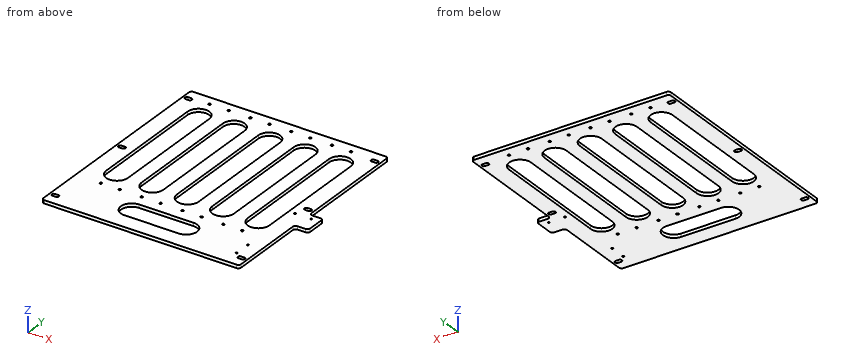
from build123d import *

# Parameters (mm, degrees)
SKETCH_1_W             = 363
SKETCH_1_H             = 403
EXTRUDE_1_DEPTH        = 6
FILLET_1_R             = 5
SKETCH_3_R             = 3.5
CUT_EXTRUDE_2_DEPTH    = 10
HOLE_WIZARD_M5_1_D     = 4.2
HOLE_WIZARD_M5_1_DEPTH = 12.4
HOLE_WIZARD_M5_1_TIP   = 1.2618073
CUT_EXTRUDE_3_DEPTH    = 10
CUT_EXTRUDE_4_DEPTH    = 10
CUT_EXTRUDE_5_DEPTH    = 10
HOLE_WIZARD_M4_1_D     = 3.3
HOLE_WIZARD_M4_1_DEPTH = 10.1
HOLE_WIZARD_M4_1_TIP   = 0.991420021
SKETCH_11_W            = 25
SKETCH_11_H            = 40
EXTRUDE_2_DEPTH        = 6
HOLE_WIZARD_M4_2_D     = 3.3
HOLE_WIZARD_M4_2_DEPTH = 10.1
HOLE_WIZARD_M4_2_TIP   = 0.991420021
FILLET_2_R             = 5


with BuildPart() as part:
    # Sketch 1 → 凸台-拉伸1 (new body)
    with BuildSketch(Plane.XY):
        Rectangle(SKETCH_1_W, SKETCH_1_H)
    extrude(amount=EXTRUDE_1_DEPTH)

    # 圆角1
    fillet_1_edges = [part.edges().sort_by_distance(p)[0] for p in [
        (181.5, -201.5, 3),
        (-181.5, -201.5, 3),
        (-181.5, 201.5, 3),
        (181.5, 201.5, 3),
    ]]
    fillet(fillet_1_edges, radius=FILLET_1_R)

    # 草图3 → 切除-拉伸2 (cut)
    with BuildSketch(Plane.XY.offset(6)):
        with Locations((-171, -180)):
            Circle(SKETCH_3_R)
        with Locations((-171, 180)):
            Circle(SKETCH_3_R)
        with Locations((-171, 0)):
            Circle(SKETCH_3_R)
        with Locations((171, 0)):
            Circle(SKETCH_3_R)
        with Locations((171, 180)):
            Circle(SKETCH_3_R)
        with Locations((171, -180)):
            Circle(SKETCH_3_R)
    extrude(amount=-CUT_EXTRUDE_2_DEPTH, mode=Mode.SUBTRACT)

    # M5 螺纹孔1
    with Locations(Plane.XY.offset(6)):
        with Locations((-135, -110), (-100, -110), (-135, 184), (-100, 184), (-60, -110), (-25, -110), (-60, 184), (-25, 184), (15, -110), (50, -110), (15, 184), (50, 184), (90, -110), (125, -110), (90, 184), (125, 184)):
            Hole(HOLE_WIZARD_M5_1_D / 2, depth=HOLE_WIZARD_M5_1_DEPTH)
            with Locations((0, 0, -(HOLE_WIZARD_M5_1_DEPTH + HOLE_WIZARD_M5_1_TIP / 2))):  # 118° drill point
                Cone(0, HOLE_WIZARD_M5_1_D / 2, HOLE_WIZARD_M5_1_TIP, mode=Mode.SUBTRACT)

    # 草图6 → 切除-拉伸3 (cut)
    with BuildSketch(Plane.XY.offset(6)):
        with BuildLine():
            Line((-174, 183.5), (-168, 183.5))
            ThreePointArc((-168, 183.5), (-164.5, 180), (-168, 176.5))
            Line((-168, 176.5), (-174, 176.5))
            ThreePointArc((-174, 176.5), (-177.5, 180), (-174, 183.5))
        make_face()
        with BuildLine():
            Line((168, 183.5), (174, 183.5))
            ThreePointArc((174, 183.5), (177.5, 180), (174, 176.5))
            Line((174, 176.5), (168, 176.5))
            ThreePointArc((168, 176.5), (164.5, 180), (168, 183.5))
        make_face()
        with BuildLine():
            Line((168, 3.5), (174, 3.5))
            ThreePointArc((174, 3.5), (177.5, 0), (174, -3.5))
            Line((174, -3.5), (168, -3.5))
            ThreePointArc((168, -3.5), (164.5, 0), (168, 3.5))
        make_face()
        with BuildLine():
            Line((168, -176.5), (174, -176.5))
            ThreePointArc((174, -176.5), (177.5, -180), (174, -183.5))
            Line((174, -183.5), (168, -183.5))
            ThreePointArc((168, -183.5), (164.5, -180), (168, -176.5))
        make_face()
        with BuildLine():
            Line((-174, 3.5), (-168, 3.5))
            ThreePointArc((-168, 3.5), (-164.5, 0), (-168, -3.5))
            Line((-168, -3.5), (-174, -3.5))
            ThreePointArc((-174, -3.5), (-177.5, 0), (-174, 3.5))
        make_face()
        with BuildLine():
            Line((-174, -176.5), (-168, -176.5))
            ThreePointArc((-168, -176.5), (-164.5, -180), (-168, -183.5))
            Line((-168, -183.5), (-174, -183.5))
            ThreePointArc((-174, -183.5), (-177.5, -180), (-174, -176.5))
        make_face()
    extrude(amount=-CUT_EXTRUDE_3_DEPTH, mode=Mode.SUBTRACT)

    # 草图7 → 切除-拉伸4 (cut)
    with BuildSketch(Plane.XY.offset(6)):
        with BuildLine():
            Line((-50, -131.5), (50, -131.5))
            ThreePointArc((50, -131.5), (70, -151.5), (50, -171.5))
            Line((50, -171.5), (-50, -171.5))
            ThreePointArc((-50, -171.5), (-70, -151.5), (-50, -131.5))
        make_face()
    extrude(amount=-CUT_EXTRUDE_4_DEPTH, mode=Mode.SUBTRACT)

    # 草图8 → 切除-拉伸5 (cut)
    with BuildSketch(Plane.XY.offset(6)):
        with BuildLine():
            Line((20, 146.5), (20, -73.5))
            ThreePointArc((20, -73.5), (0, -93.5), (-20, -73.5))
            Line((-20, -73.5), (-20, 146.5))
            ThreePointArc((-20, 146.5), (0, 166.5), (20, 146.5))
        make_face()
        with BuildLine():
            Line((85, 146.5), (85, -73.5))
            ThreePointArc((85, -73.5), (65, -93.5), (45, -73.5))
            Line((45, -73.5), (45, 146.5))
            ThreePointArc((45, 146.5), (65, 166.5), (85, 146.5))
        make_face()
        with BuildLine():
            Line((150, 146.5), (150, -73.5))
            ThreePointArc((150, -73.5), (130, -93.5), (110, -73.5))
            Line((110, -73.5), (110, 146.5))
            ThreePointArc((110, 146.5), (130, 166.5), (150, 146.5))
        make_face()
        with BuildLine():
            Line((-150, 146.5), (-150, -73.5))
            ThreePointArc((-150, -73.5), (-130, -93.5), (-110, -73.5))
            Line((-110, -73.5), (-110, 146.5))
            ThreePointArc((-110, 146.5), (-130, 166.5), (-150, 146.5))
        make_face()
        with BuildLine():
            Line((-85, 146.5), (-85, -73.5))
            ThreePointArc((-85, -73.5), (-65, -93.5), (-45, -73.5))
            Line((-45, -73.5), (-45, 146.5))
            ThreePointArc((-45, 146.5), (-65, 166.5), (-85, 146.5))
        make_face()
    extrude(amount=-CUT_EXTRUDE_5_DEPTH, mode=Mode.SUBTRACT)

    # M4 螺纹孔1
    with Locations(Plane.XY.offset(6)):
        with Locations((156.5, -171.5), (156.5, -141.5)):
            Hole(HOLE_WIZARD_M4_1_D / 2, depth=HOLE_WIZARD_M4_1_DEPTH)
            with Locations((0, 0, -(HOLE_WIZARD_M4_1_DEPTH + HOLE_WIZARD_M4_1_TIP / 2))):  # 118° drill point
                Cone(0, HOLE_WIZARD_M4_1_D / 2, HOLE_WIZARD_M4_1_TIP, mode=Mode.SUBTRACT)

    # 草图11 → 凸台-拉伸2 (add)
    with BuildSketch(Plane.XY.offset(6)):
        with Locations((194, -31.5)):
            Rectangle(SKETCH_11_W, SKETCH_11_H)
    extrude(amount=-EXTRUDE_2_DEPTH)

    # M4 螺纹孔2
    with Locations(Plane.XY.offset(6)):
        with Locations((161.5, -21.5), (191.5, -21.5)):
            Hole(HOLE_WIZARD_M4_2_D / 2, depth=HOLE_WIZARD_M4_2_DEPTH)
            with Locations((0, 0, -(HOLE_WIZARD_M4_2_DEPTH + HOLE_WIZARD_M4_2_TIP / 2))):  # 118° drill point
                Cone(0, HOLE_WIZARD_M4_2_D / 2, HOLE_WIZARD_M4_2_TIP, mode=Mode.SUBTRACT)

    # 圆角2
    fillet_2_edges = [part.edges().sort_by_distance(p)[0] for p in [
        (181.5, -51.5, 3),
        (181.5, -11.5, 3),
        (206.5, -11.5, 3),
        (206.5, -51.5, 3),
    ]]
    fillet(fillet_2_edges, radius=FILLET_2_R)


solid = part.part
Input: part model. Units: mm. Frame: model coordinates. Give positions to 0.01 mm unless a question says otherwise; leave off trailing zeros. Write each loop counter-clockwise with the first axis right and the second up, starting at its lowest first coordinate (ties: lowest second). Pieces come first, ordered by that corner, then holes.
Q1. Section A-A, the plane y = 129.5. Output: boundary loops of the cut face in (x, z).
Q2. Material intervals for probe 1 along X at (y, z) = (17.5, 5.5); probe 2 along Y at (x, z) = (-100, 4.2); probe 3 along Y at (x, z) = (65, 2.35), sorted ascending.
Q3. Section C-C, the plane x = 65. Output: boundary loops of the cut face in (y, z), plus the area to 3 significant figures.
Q4. First-contact query: P1, Ø1.8, axis at y = 32.5, z = 3.5, coming from the +X side; P2, Ø3, axis at x = 194.5, z = 3, coming from the -Y side; P3, Ø5.5, axis at x = -100, y = 184, coming from the +Z side. Flat tips, straight axial feed; report the tip coordinate or a pass-through.
Q5. Section B-B, the plane x = -119. Output: boundary loops of the cut face in (y, z).
Q6. Section D-D, the plane z = 3.1. State how many separate pieces and enclosed holes the cut face has, plus the area to 3 significant figures.
Filled in:
1. outline: (-181.5, 0) - (-150, 0) - (-150, 6) - (-181.5, 6) - close; (-110, 0) - (-85, 0) - (-85, 6) - (-110, 6) - close; (-45, 0) - (-20, 0) - (-20, 6) - (-45, 6) - close; (20, 0) - (45, 0) - (45, 6) - (20, 6) - close; (85, 0) - (110, 0) - (110, 6) - (85, 6) - close; (150, 0) - (181.5, 0) - (181.5, 6) - (150, 6) - close
2. probe 1: x = -181.5 to -150, -110 to -85, -45 to -20, 20 to 45, 85 to 110, 150 to 181.5
2. probe 2: y = -201.5 to -112.1, -107.9 to 181.9, 186.1 to 201.5
2. probe 3: y = -201.5 to -164.73, -138.27 to -93.5, 166.5 to 201.5
3. outline: (-201.5, 0) - (-164.73, 0) - (-164.73, 6) - (-201.5, 6) - close; (-138.27, 0) - (-93.5, 0) - (-93.5, 6) - (-138.27, 6) - close; (166.5, 0) - (201.5, 0) - (201.5, 6) - (166.5, 6) - close
3. area: 699 mm2
4. P1: stops at x = 181.5
4. P2: stops at y = -51.5
4. P3: stops at z = 6
5. outline: (-201.5, 0) - (-90.2, 0) - (-90.2, 6) - (-201.5, 6) - close; (163.2, 0) - (201.5, 0) - (201.5, 6) - (163.2, 6) - close
6. separate pieces: 1
6. enclosed holes: 32
6. area: 91,000 mm2
